```python
from build123d import *

# Parameters (mm, degrees)
SKETCH001_W  = 67
SKETCH001_H  = 53
PAD001_DEPTH = 15
SKETCH002_W  = 11
SKETCH002_H  = 12
PAD002_DEPTH = 10
SKETCH003_W  = 9
SKETCH003_H  = 11
PAD003_DEPTH = 10
SKETCH_W     = 69
SKETCH_H     = 55
PAD_DEPTH    = 15


with BuildPart() as body001:
    # Sketch001 → Pad001 (new body)
    with BuildSketch(Plane.XY):
        with Locations((-27.160627, -58.233018)):
            Rectangle(SKETCH001_W, SKETCH001_H)
    extrude(amount=PAD001_DEPTH)


with BuildPart() as body001_1:
    # Body001 placement: moved
    add(body001.part.moved(Location((30, 59, 1))))


with BuildPart() as body002:
    # Sketch002 → Pad002 (new body)
    with BuildSketch(Plane.YZ):
        with Locations((5.5, 6)):
            Rectangle(SKETCH002_W, SKETCH002_H)
    extrude(amount=PAD002_DEPTH)


with BuildPart() as body002_1:
    # Body002 placement: moved
    add(body002.part.moved(Location((-32, 4, 4))))


with BuildPart() as body003:
    # Sketch003 → Pad003 (new body)
    with BuildSketch(Plane.XY):
        with Locations((-41.905017, -12.711954)):
            Rectangle(SKETCH003_W, SKETCH003_H)
    extrude(amount=PAD003_DEPTH)


with BuildPart() as body003_1:
    # Body003 placement: moved
    add(body003.part.moved(Location((9, -2, 4))))


with BuildPart() as body:
    # Sketch → Pad (new body)
    with BuildSketch(Plane.XY):
        with Locations((2.865111, 0.748495)):
            Rectangle(SKETCH_W, SKETCH_H)
    extrude(amount=PAD_DEPTH)

    # Boolean: cut Body001
    add(body001_1.part, mode=Mode.SUBTRACT)

    # Boolean001: cut Body002
    add(body002_1.part, mode=Mode.SUBTRACT)

    # Boolean002: cut Body003
    add(body003_1.part, mode=Mode.SUBTRACT)


solid = body.part
```
Input: part model. Units: mm. Frame: model coordinates. A direction names the side the tool comes from. Coordinates: 2 decimals unless noted, no trailing zeros. Write each loop counter-clockwise with the first axis right and the second up, starting at its lowest first coordinate (ties: lowest second). Pieces come first, ordered by that corner, then holes. Notation, with made-up numbers: (54, 66) - (85, 66) arc R13 ccw to (85, 87) - close; hole circle Ø2 at (-38.75, 68). An arc over 180 degrees is marked (long way). Put each result on its own line as item: value. Start each with the question number.
1) Cut plane B-B (y = -17.5). Return the cut outline in (x, z).
2) Cut plane D-D (y = 11). Return the cut outline in (x, z).
3) Contact query for flat-ended pins moving along their axis: pin 1 (3 mm diameter, centred on x = 6.5, y = 7, fed in from +Z); pin 2 (4 mm diameter, centred on x = 9, y = -17.5, fed in from -Z); pin 3 (1.1 mm diameter, centred on x = -31, y = 8, fed in from +Z). Output: stop coordinate, or through.
4) Ray query, L1, parallel to X at y = -17, z = 2; L2, parallel to Y at x = -16, z = 12; L3, parallel to Z at x = 6.5, y = 1. Return the intervals inside material, ascending.
5) Mould query, pull axis Y, two halves, no side actions, for faces 3 (the face through (-31.635, 0, 7)), 4 (the face through (36.339, 0, 8)), 5 (the face through (2, 28.248, 7)). Classes: pulls with the +Y half, pulls with the -Y half, needs draft (parallel to the pull), parting line crosses it, or undercut.
6) Reachability of faces 1 (the face through (2, 1, 0)), 2 (the face through (2, -25.733, 8)) from +Z, -Z, +X, -X, +Y, -Y: full face, straight path, thin tool, end or side. Return the list, or none.
7) Cut plane C-C (z = 11.5). Return the cut outline in (x, y), plus the area to 3 significant figures.
8) Cut plane A-A (z = 2.5). Return the cut outline in (x, y).
Resolved:
1. outline: (-31.63, 0) - (37.37, 0) - (37.37, 15) - (36.34, 15) - (36.34, 1) - (-30.66, 1) - (-30.66, 4) - (-31.63, 4) - close; (-31.63, 14) - (-30.66, 14) - (-30.66, 15) - (-31.63, 15) - close
2. outline: (-31.63, 0) - (37.37, 0) - (37.37, 15) - (36.34, 15) - (36.34, 1) - (-30.66, 1) - (-30.66, 4) - (-31.63, 4) - close
3. pin 1: stops at z = 1
3. pin 2: stops at z = 0
3. pin 3: stops at z = 4
4. L1: x = -31.63 to -30.66, 36.34 to 37.37
4. L2: y = -26.75 to -25.73, 27.27 to 28.25
4. L3: z = 0 to 1
5. face 3: needs draft
5. face 4: undercut
5. face 5: pulls with the +Y half
6. face 1: -Z, +X, -X, +Y, -Y
6. face 2: +Z
7. outline: (-31.63, -26.75) - (37.37, -26.75) - (37.37, 28.25) - (-31.63, 28.25) - (-31.63, 15) - (-30.66, 15) - (-30.66, 27.27) - (36.34, 27.27) - (36.34, -25.73) - (-30.66, -25.73) - (-30.66, -20.21) - (-31.63, -20.21) - close; (-31.63, -9.21) - (-30.66, -9.21) - (-30.66, 4) - (-31.63, 4) - close
7. area: 223 mm2
8. outline: (-31.63, -26.75) - (37.37, -26.75) - (37.37, 28.25) - (-31.63, 28.25) - close; hole (-30.66, -25.73) - (36.34, -25.73) - (36.34, 27.27) - (-30.66, 27.27) - close
